Build history of the part. All positions in model axes, mm. Give positions to 0.01 mm unless a question says otherwise; leave off trailing zeros. One line per item, written item: value. Start each with the question number.
from build123d import *

# Parameters (mm, degrees)
SKETCH_1_W          = 720
SKETCH_1_H          = 520
EXTRUDE_1_DEPTH     = 5
CUT_EXTRUDE_1_DEPTH = 445.100213916
SKETCH_3_R          = 2.5
CUT_EXTRUDE_2_DEPTH = 445.100213916
FILLET_1_R          = 5


with BuildPart() as part:
    # 草图1 → 凸台-拉伸1 (new body)
    with BuildSketch(Plane.XY):
        Rectangle(SKETCH_1_W, SKETCH_1_H)
    extrude(amount=EXTRUDE_1_DEPTH)

    # 草图2 → 切除-拉伸1 (cut, through all)
    with BuildSketch(Plane.XY.offset(5)):
        Polygon((340, -240), (340, -200), (360, -200), (360, -260), (300, -260), (300, -240), align=None)
        Polygon((340, 240), (300, 240), (300, 260), (360, 260), (360, 200), (340, 200), align=None)
        Polygon((-340, 240), (-340, 200), (-360, 200), (-360, 260), (-300, 260), (-300, 240), align=None)
        Polygon((-340, -240), (-300, -240), (-300, -260), (-360, -260), (-360, -200), (-340, -200), align=None)
    extrude(amount=-CUT_EXTRUDE_1_DEPTH, mode=Mode.SUBTRACT)

    # 草图3 → 切除-拉伸2 (cut, through all)
    with BuildSketch(Plane.XY.offset(5)):
        with Locations((350, 180)):
            Circle(SKETCH_3_R)
        with Locations((280, 250)):
            Circle(SKETCH_3_R)
        with Locations((-280, 250)):
            Circle(SKETCH_3_R)
        with Locations((-350, 180)):
            Circle(SKETCH_3_R)
        with Locations((-350, -180)):
            Circle(SKETCH_3_R)
        with Locations((-280, -250)):
            Circle(SKETCH_3_R)
        with Locations((350, -180)):
            Circle(SKETCH_3_R)
        with Locations((280, -250)):
            Circle(SKETCH_3_R)
    extrude(amount=-CUT_EXTRUDE_2_DEPTH, mode=Mode.SUBTRACT)

    # 圆角1
    fillet_1_edges = [part.edges().sort_by_distance(p)[0] for p in [
        (-360, -200, 2.5),
        (-340, -200, 2.5),
        (-340, -240, 2.5),
        (-300, -240, 2.5),
        (-300, -260, 2.5),
        (-300, 260, 2.5),
        (-300, 240, 2.5),
        (-340, 240, 2.5),
        (-340, 200, 2.5),
        (-360, 200, 2.5),
        (360, 200, 2.5),
        (340, 200, 2.5),
        (340, 240, 2.5),
        (300, 240, 2.5),
        (300, 260, 2.5),
        (300, -260, 2.5),
        (300, -240, 2.5),
        (340, -240, 2.5),
        (340, -200, 2.5),
        (360, -200, 2.5),
    ]]
    fillet(fillet_1_edges, radius=FILLET_1_R)


solid = part.part
1) Slice it at A-A (z = 3.15). State how many separate pieces and enclosed holes the cut face has, plus the area to 3 significant figures.
2) Drop flat-ended pins along their axis: P1, Ø6, axis at x = 247, y = -128, coming from the -Z side; P2, Ø2.5, axis at y = 251.5, z = 3, coming from the +X side; P3, Ø2.5, axis at x = -347.5, z = 2.5, coming from the -Y side. Give the stop position or say it passes through.
3) Drill centre lines: line 1 (Y direction, x = 280, z = 3.6); line 2 (Y direction, x = 350, z = 1.95); line 3 (X direction, y = 180, z = 3.25). Where is each one in solid material? Low to high.
Results list:
1. separate pieces: 1
1. enclosed holes: 8
1. area: 366,000 mm²
2. P1: stops at z = 0
2. P2: stops at x = 300
2. P3: stops at y = -200
3. line 1: y = -260 to -252.5, -247.5 to 247.5, 252.5 to 260
3. line 2: y = -200 to -182.5, -177.5 to 177.5, 182.5 to 200
3. line 3: x = -360 to -352.5, -347.5 to 347.5, 352.5 to 360
